Design review of the part shown in the three views and the two pictorial views. Dimensions are in mm from the part's minimum x, y and z. A direction names the side the tool comes from. Coordinates: 2 decimals unless noted, no trailing zeros. Write each loop counter-clockwise with the first axis right and the second up, starting at its lowest first coordinate (ties: lowest second). Pieces come first, ordered by that corner, then holes. Notation, with made-up numbers: (89.5, 21) -> (107.5, 21) arc R33 cw to (107.5, 49) -> close; hole circle Ø5 at (62, 42). An arc over 180 degrees is marked (long way). Write each question's results on one line, items separated by ' | '.
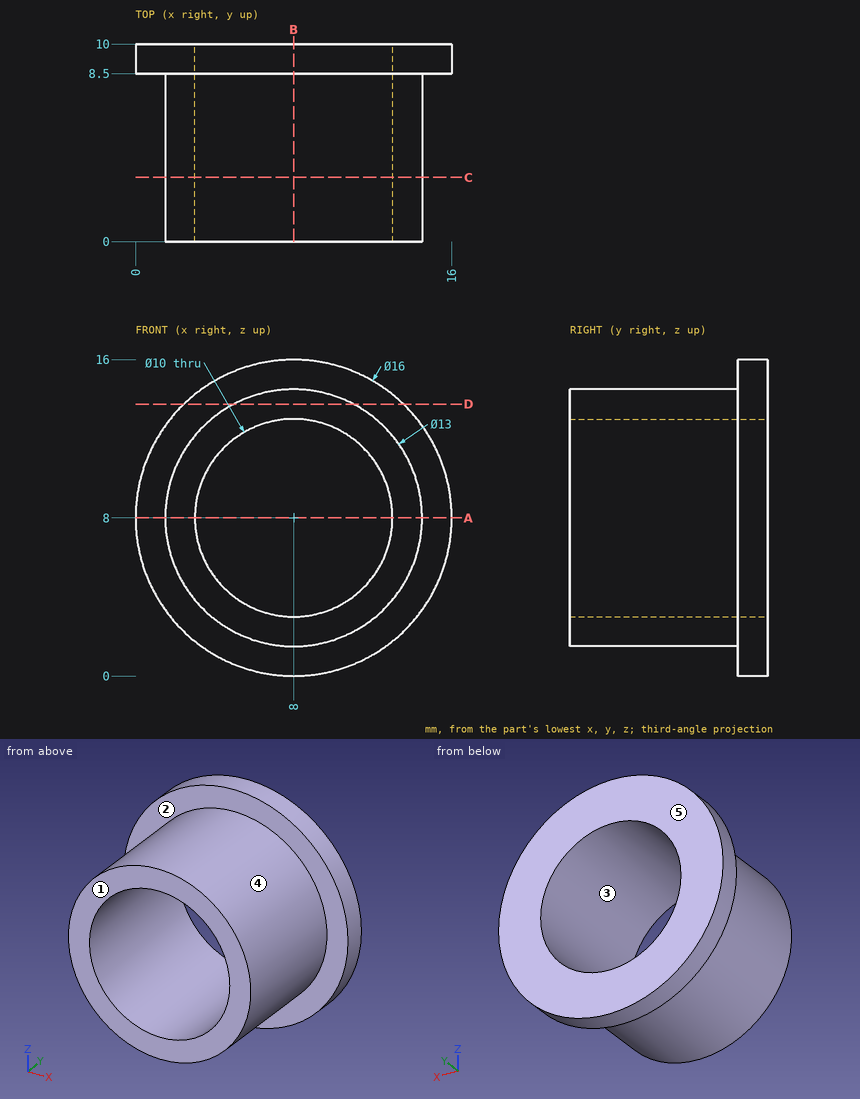
Q1. Add section B-B (x = 8). Write out the cut boundary in (y, z), plus the area to 3 significant figures.
Solution:
outline: (0, 1.5) -> (8.5, 1.5) -> (8.5, 0) -> (10, 0) -> (10, 3) -> (0, 3) -> close; (0, 13) -> (10, 13) -> (10, 16) -> (8.5, 16) -> (8.5, 14.5) -> (0, 14.5) -> close | area: 34.5 mm²
Q2. Clearance check with flat-ended pins moving along their axes: P1, Ø1, axis at x = 10, z = 12.5, coming from the -Y side; P2, Ø1.5, axis at x = 3.5, y = 5, coming from the -Z side; P3, Ø1, axis at x = 5.5, y = 7, coming from the +Z side; P4, Ø4, axis at x = 13, y = 1, coming from the +Z side. State where each tip first meets the part, or that it passes through.
Solution:
P1: y = 0 | P2: z = 2.69 | P3: z = 14.18 | P4: z = 13.77
Q3. Add section A-A (z = 8). Write out the cut boundary in (x, y).
Solution:
outline: (0, 8.5) -> (1.5, 8.5) -> (1.5, 0) -> (3, 0) -> (3, 10) -> (0, 10) -> close; (13, 0) -> (14.5, 0) -> (14.5, 8.5) -> (16, 8.5) -> (16, 10) -> (13, 10) -> close
Q4. Add section D-D (z = 13.75). Write out the cut boundary in (x, y), plus the area to 3 significant figures.
Solution:
outline: (2.44, 8.5) -> (4.97, 8.5) -> (4.97, 0) -> (11.03, 0) -> (11.03, 8.5) -> (13.56, 8.5) -> (13.56, 10) -> (2.44, 10) -> close | area: 68.2 mm²
Q5. Draft analysis for pull direction X (two halves, no side actions). For the marked faces 3, 4 and 5, state which applies: pulls with the +X half, pulls with the -X half, needs draft (parallel to the pull), parting line crosses it, or undercut.
Solution:
face 3: undercut | face 4: parting line crosses it | face 5: needs draft
Q6. For line 1 (X direction, y = 5, z = 8); line 2 (Z direction, x = 10.75, y = 8); line 3 (X direction, y = 9.5, z = 11.75), list the stretches that pass through material, from the lowest coordinate up. Write a range as from..to.
Solution:
line 1: 1.5..3, 13..14.5 | line 2: 2.11..3.82, 12.18..13.89 | line 3: 0.93..4.69, 11.31..15.07
Q7. Machinability: for the marked faces 1 and 2, which of the approach directions +Z, -Z, +X, -X, +Y, -Y give a long, thin tool a straight path to every point of the face, cutting with its end or side? Answer none if there is none.
Solution:
face 1: +Z, -Z, +X, -X, -Y | face 2: -Y
Q8. Add section C-C (y = 3.25). Write out the cut boundary in (x, z), plus the area to 3 significant figures.
Solution:
outline: circle Ø13 at (8, 8); hole circle Ø10 at (8, 8) | area: 54.2 mm²
